from build123d import *

# Parameters (mm, degrees)
F0_W     = 75
F0_H     = 75
F1_DEPTH = 5
F2_W     = 5
F2_H     = 5
F2_W_2   = 3.2
F2_H_2   = 3.2
F2_W_3   = 61.8
F2_H_3   = 61.8
F3_DEPTH = 70
F4_R     = 2
F5_W     = 3.2
F5_H     = 3.2
F6_DEPTH = 75


# Not quite as in the source:
# - a feature names something its author has since deleted; it is built from what else it names


with BuildPart() as f1:
    # F0 (on Top) → F1 (new body)
    with BuildSketch(Plane.XY):
        Rectangle(F0_W, F0_H)
    extrude(amount=F1_DEPTH)

    # F2 (on face) → F3 (join)
    with BuildSketch(Plane.XY.offset(5)):
        with Locations((-35, 35)):
            Rectangle(F2_W, F2_H)
        with Locations((-30.9, 35)):
            Rectangle(F2_W_2, F2_H)
        with Locations((-35, 30.9)):
            Rectangle(F2_W, F2_H_2)
        with Locations((-26.8, 35)):
            Rectangle(F2_W, F2_H)
        with Locations((-35, 26.8)):
            Rectangle(F2_W, F2_H)
        with Locations((-30.9, 26.8)):
            Rectangle(F2_W_2, F2_H)
        with Locations((-26.8, 30.9)):
            Rectangle(F2_W, F2_H_2)
        with Locations((6.6, 35)):
            Rectangle(F2_W_3, F2_H)
        with Locations((-35, -6.6)):
            Rectangle(F2_W, F2_H_3)
        with Locations((-26.8, 26.8)):
            Rectangle(F2_W, F2_H)
        with Locations((-26.8, -6.6)):
            Rectangle(F2_W, F2_H_3)
        with Locations((6.6, 26.8)):
            Rectangle(F2_W_3, F2_H)
    extrude(amount=F3_DEPTH)

    # F4
    f4_edges = [f1.edges().sort_by_distance(p)[0] for p in [
        (0, -37.5, 0),
        (37.5, 0, 0),
        (0, 37.5, 0),
        (-37.5, 0, 0),
        (-37.5, 37.5, 37.5),
        (-37.5, 0, 75),
        (-37.5, -37.5, 37.5),
        (37.5, 37.5, 37.5),
        (0, 37.5, 75),
        (-24.3, -6.6, 5),
        (6.6, 24.3, 5),
        (37.5, -6.6, 5),
        (6.6, -37.5, 5),
        (-24.3, 24.3, 40),
        (-24.3, -37.5, 40),
        (37.5, 24.3, 40),
    ]]
    fillet(f4_edges, radius=F4_R)

    # F5 (on face) → F6 (join, through all)
    with BuildSketch(Plane.XY.offset(75)):
        with Locations((-30.9, 30.9)):
            Rectangle(F5_W, F5_H)
    extrude(amount=-F6_DEPTH)


solid = f1.part
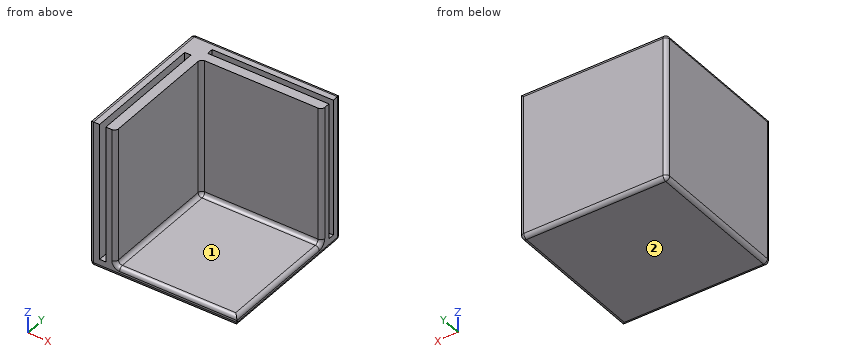
CAD build for the part. Positions are in the model's coordinates, mm. Face numbers are marked on the shaded views. A direction names the side the tool comes from. Coordinates: 2 decimals unless noted, no trailing zeros. Loops run counter-clockwise (first coordinate to the right, second up) from the corner with the lowest first, then second, coordinate; pieces in that order, holes last. Notation, with made-up numbers: (-8.75, 82) - (15.25, 82) arc R32 ccw to (15.25, 108) - close; hole circle Ø7 at (23, 29.5). An arc over 180 degrees is marked (long way). Write item = value, one per line. Start each with the question number.
Q1. Flat gauge pins, fed straight in: pin 1 Ø1 at (y, z) = (-1, 65) entering from +X; pin 2 Ø1.6 at (x, y) = (0, 31) entering from +Z; pin 3 Ø3.5 at (y, z) = (31, 38.5) entering from +X; pin 4 Ø2.5 at (x, z) = (-31, 38.5) entering from -Y. Where does each tip first touch, or does it go through?
Q2. Cut at B-B, the plane x = 33.5. List the corners of the cut face in (y, z).
Q3. Cut at A-A, the plane z = 16. List the corners of the cut face in (x, y), then the cut area to 3 significant figures.
Q4. Cut at C-C, the plane y = -20. List the corners of the cut face in (x, z), then the cut area to 3 significant figures.
Q5. Drill centre lines: L1, parallel to Y at x = -16, z = 48; L2, parallel to X at y = 8, z = 52.5; L3, parallel to Z at x = 24.5, y = -11. Where is each one in solid material? Low to high.
Q6. Which spindle directions (+Z, -Z, +X, -X, +Y, -Y) get a long thin tool onto all of the face, cutting with end or side? Do the marked faces 1 and 2. Say none if no direction does.
Computed:
q1.pin_1 = -24.3
q1.pin_2 = 5
q1.pin_3 = 37.5
q1.pin_4 = 24.3
q2.outline = (-37.5, 2) arc R2 ccw to (-35.5, 0) - (35.5, 0) arc R2 ccw to (37.5, 2) - (37.5, 73) arc R2 ccw to (35.5, 75) - (32.5, 75) - (32.5, 5) - (29.3, 5) - (29.3, 75) - (24.3, 75) - (24.3, 7) arc R2 cw to (22.3, 5) - (-35.5, 5) arc R2 ccw to (-37.5, 3) - close
q3.outline = (-37.5, -35.5) arc R2 ccw to (-35.5, -37.5) - (-32.5, -37.5) - (-32.5, 24.3) - (-29.3, 24.3) - (-29.3, -37.5) - (-26.3, -37.5) arc R2 ccw to (-24.3, -35.5) - (-24.3, 22.3) arc R2 cw to (-22.3, 24.3) - (35.5, 24.3) arc R2 ccw to (37.5, 26.3) - (37.5, 29.3) - (-24.3, 29.3) - (-24.3, 32.5) - (37.5, 32.5) - (37.5, 35.5) arc R2 ccw to (35.5, 37.5) - (-35.5, 37.5) arc R2 ccw to (-37.5, 35.5) - close
q3.area = 1,410 mm²
q4.outline = (-37.5, 2) arc R2 ccw to (-35.5, 0) - (35.5, 0) arc R2 ccw to (37.5, 2) - (37.5, 3) arc R2 ccw to (35.5, 5) - (-22.3, 5) arc R2 cw to (-24.3, 7) - (-24.3, 75) - (-29.3, 75) - (-29.3, 5) - (-32.5, 5) - (-32.5, 75) - (-35.5, 75) arc R2 ccw to (-37.5, 73) - close
q4.area = 1,070 mm²
q5.L1 = 24.3 to 29.3, 32.5 to 37.5
q5.L2 = -37.5 to -32.5, -29.3 to -24.3
q5.L3 = 0 to 5
q6.face_1 = +Z, +X, -Y
q6.face_2 = -Z, +X, -X, +Y, -Y
